The model under review builds one solid part; all positions refer to its coordinate system, in mm. Round coordinates to 2 decimals unless told otherwise and drop trailing zeros. Write each loop counter-clockwise with the first axis right and the second up, starting at its lowest first coordinate (ties: lowest second). Pieces come first, ordered by that corner, then holes. Notation, with made-up numbers: M 12,36.25 L 56,36.25 A37 ccw 56,72.25 Z; hole C 64,-33.75 d7. An arc over 180 degrees is marked long. Write item = value, one per line. Start each with the question number.
Item 1: Take a section at D-D, the plane x = 18. Give the boundary of the cut face in (y, z), plus the area to 3 significant figures.
Item 2: Take a section at A-A, the plane x = 0. Give the boundary of the cut face in (y, z), plus the area to 3 significant figures.
Item 3: To check wall thickness, follow line 1 along X through (y, z) = (-2.9, 11); line 2 along X through (y, z) = (-3.15, 3.5); line 3 along Z through (x, y) = (-78, -1.1). State the ranges of each line that lie inside material, in increasing order.
Item 4: Take a section at B-B, the plane x = -76.5. Give the boundary of the cut face in (y, z), plus the area to 3 significant figures.
Item 5: Take a section at C-C, the plane y = -3.75. Give the number of separate pieces and of enclosed holes in the cut face, plus the area to 3 significant figures.
Item 6: For pin 1 Ø1.5 at (x, y) = (-17.5, -3.5) entering from -Z; pin 2 Ø8 at (x, z) = (0, 0) entering from -Y; pin 3 Ø1.5 at (x, y) = (-72.5, -3.5) entering from +Z; pin 4 Ø1 at (x, y) = (-86.5, -3.5) entering from +Z, all flat-tipped, find the tip position at first contact; note any pin that passes through.
from build123d import *

# Parameters (mm, degrees)
SKETCH_2_R          = 5
EXTRUDE_1_DEPTH     = 5
CUT_EXTRUDE_1_DEPTH = 92.187134051
FILLET_1_R          = 2.8
FILLET_2_R          = 2.8
FILLET_3_R          = 10
FILLET_4_R          = 5
FILLET_5_R          = 2.5
FILLET_6_R          = 10


with BuildPart() as part:
    # 草图2 → 凸台-拉伸1 (new body)
    # profile 1 of 2: a face of its own
    with BuildSketch(Plane(origin=(0, 0, 0), x_dir=(1, 0, 0), z_dir=(0, 1, 0))):
        with BuildLine():
            Line((-55.8, 9.5), (-65.4, 9.5))
            ThreePointArc((-65.4, 9.5), (-60.625065445, 8.212794896), (-57.144093024, 4.7))
            Line((-57.144093024, 4.7), (-49.644093024, 4.7))
            Line((-49.644093024, 4.7), (-47.528169255, -7.3))
            Line((-47.528169255, -7.3), (-32.828169255, -7.3))
            Line((-32.828169255, -7.3), (-26.77268488, -4.8))
            Line((-26.77268488, -4.8), (-8.77268488, -4.8))
            ThreePointArc((-8.77268488, -4.8), (-3.040245716, -9.526641905), (4.370469962, -8.994386711))
            ThreePointArc((4.370469962, -8.994386711), (20.084939282, -6.943193169), (33.875265504, -14.75208833))
            Line((33.875265504, -14.75208833), (44.771139737, -26.853182613))
            Line((44.771139737, -26.853182613), (62.606615548, -10.794048061))
            Line((62.606615548, -10.794048061), (51.23139524, 1.839413972))
            Line((51.23139524, 1.839413972), (39, -1.933246956))
            Line((39, -1.933246956), (9.777013859, 2.1))
            ThreePointArc((9.777013859, 2.1), (1.554340892, 9.878462653), (-8.659704384, 5.000951907))
            Line((-8.659704384, 5.000951907), (-26.659704384, 5.000951907))
            Line((-26.659704384, 5.000951907), (-34.031178231, 15.096068218))
            Line((-34.031178231, 15.096068218), (-47.312951043, 14.4))
            Line((-47.312951043, 14.4), (-55.8, 9.5))
        make_face()
        with Locations(Location((0, 0, 0), (0, 0, 270))):
            Circle(SKETCH_2_R, mode=Mode.SUBTRACT)
    # profile 2 of 2: a face of its own
    with BuildSketch(Plane(origin=(0, 0, 0), x_dir=(1, 0, 0), z_dir=(0, 1, 0))):
        with BuildLine():
            Line((-80.324573519, -9.5), (-65.4, -9.5))
            ThreePointArc((-65.4, -9.5), (-55.9, 0), (-65.4, 9.5))
            Line((-65.4, 9.5), (-80.324573519, 9.5))
            ThreePointArc((-80.324573519, 9.5), (-81.574573519, 9.834936491), (-82.489637029, 10.75))
            Line((-82.489637029, 10.75), (-83.5, 12.5))
            Line((-83.5, 12.5), (-87, 12.5))
            Line((-87, 12.5), (-82.554402927, 4.8))
            Line((-82.554402927, 4.8), (-73.598170528, 4.8))
            Line((-73.598170528, 4.8), (-73.598170528, -4.8))
            Line((-73.598170528, -4.8), (-82.554402927, -4.8))
            Line((-82.554402927, -4.8), (-87, -12.5))
            Line((-87, -12.5), (-83.5, -12.5))
            Line((-83.5, -12.5), (-82.489637029, -10.75))
            ThreePointArc((-82.489637029, -10.75), (-81.574573519, -9.834936491), (-80.324573519, -9.5))
        make_face()
        with Locations(Location((-65.4, 0, 0), (0, 0, 270))):
            Circle(SKETCH_2_R, mode=Mode.SUBTRACT)
    extrude(amount=-EXTRUDE_1_DEPTH)

    # 草图4 → 切除-拉伸1 (cut, through all)
    with BuildSketch(Plane(origin=(0, -5, 0), x_dir=(-1, 0, 0), z_dir=(0, -1, 0))):
        Polygon((42.343817462, -21.137636493), (43.940064127, 9.320564317), (36.7, 9.7), (35.103753335, -20.75820081), align=None)
        Polygon((-48.7, -4.6), (-26.034082823, -25.008483494), (-30.885279719, -30.396283479), (-53.551196896, -9.987799985), align=None)
    extrude(amount=-CUT_EXTRUDE_1_DEPTH, mode=Mode.SUBTRACT)

    # 圆角1
    fillet_1_edges = [part.edges().sort_by_distance(p)[0] for p in [
        (-57.144093024, -2.5, -4.7),
    ]]
    fillet(fillet_1_edges, radius=FILLET_1_R)

    # 圆角2
    fillet_2_edges = [part.edges().sort_by_distance(p)[0] for p in [
        (-49.644093024, -2.5, -4.7),
    ]]
    fillet(fillet_2_edges, radius=FILLET_2_R)

    # 圆角3
    fillet_3_edges = [part.edges().sort_by_distance(p)[0] for p in [
        (-47.312951043, -2.5, -14.4),
        (-34.031178231, -2.5, -15.096068218),
        (-26.659704384, -2.5, -5.000951907),
        (-8.659704384, -2.5, -5.000951907),
        (9.777013859, -2.5, -2.1),
        (39, -2.5, 1.933246956),
        (-8.77268488, -2.5, 4.8),
        (-26.77268488, -2.5, 4.8),
        (-32.828169255, -2.5, 7.3),
    ]]
    fillet(fillet_3_edges, radius=FILLET_3_R)

    # 圆角4
    fillet_4_edges = [part.edges().sort_by_distance(p)[0] for p in [
        (51.23139524, -2.5, -1.839413972),
        (62.606615548, -2.5, 10.794048061),
    ]]
    fillet(fillet_4_edges, radius=FILLET_4_R)

    # 圆角5
    fillet_5_edges = [part.edges().sort_by_distance(p)[0] for p in [
        (44.771139737, -2.5, 26.853182613),
        (-47.528169255, -2.5, 7.3),
        (-83.5, -2.5, 12.5),
        (-83.5, -2.5, -12.5),
    ]]
    fillet(fillet_5_edges, radius=FILLET_5_R)

    # 圆角6
    fillet_6_edges = [part.edges().sort_by_distance(p)[0] for p in [
        (-55.8, -2.5, -9.5),
    ]]
    fillet(fillet_6_edges, radius=FILLET_6_R)


solid = part.part
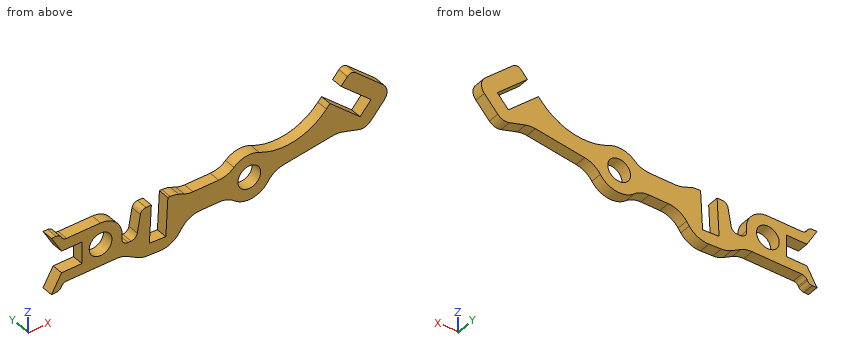
Response values:
q1.outline = M -5,-0.97 L 0,-0.97 L 0,6.63 L -5,6.63 Z
q1.area = 38.0 mm2
q2.outline = M -5,-10 L 0,-10 L 0,-5 L -5,-5 Z; M -5,5 L 0,5 L 0,10 L -5,10 Z
q2.area = 50.0 mm2
q3.line_1 = -86.13 to -82.63, 29.63 to 41.59, 52.43 to 60.51
q3.line_2 = -73.6 to -68.97, -61.83 to -56.57, -48.2 to -43.27, -36.01 to -3.57, 3.57 to 56.04
q3.line_3 = -9.5 to -4.8, 4.8 to 9.5
q4.outline = M -5,-9.5 L 0,-9.5 L 0,-4.8 L -5,-4.8 Z; M -5,4.8 L 0,4.8 L 0,9.5 L -5,9.5 Z
q4.area = 47.0 mm2
q5.separate_pieces = 1
q5.enclosed_holes = 2
q5.area = 1,720 mm2
q6.pin_1 = -5
q6.pin_2 = through
q6.pin_3 = 9.5
q6.pin_4 = 12.5
